The drawing under review shows one solid part. Ordinate dimensions are in mm from its lowest x, y, z. A direction names the side the tool comes from. Coordinates: 2 decimals unless noted, no trailing zeros. Order: outer loops, then holes, each group sorted by start corner. A loop starts at its lowest first (then second) coordinate and runs counter-clockwise, first axis right, second up. Notation, with made-up numbers: (62.5, 13.5) -> (118.5, 13.5) arc R26 cw to (118.5, 52.5) -> close; hole circle Ø10 at (67, -38). An arc over 180 degrees is marked (long way). Write item = value, one per line.
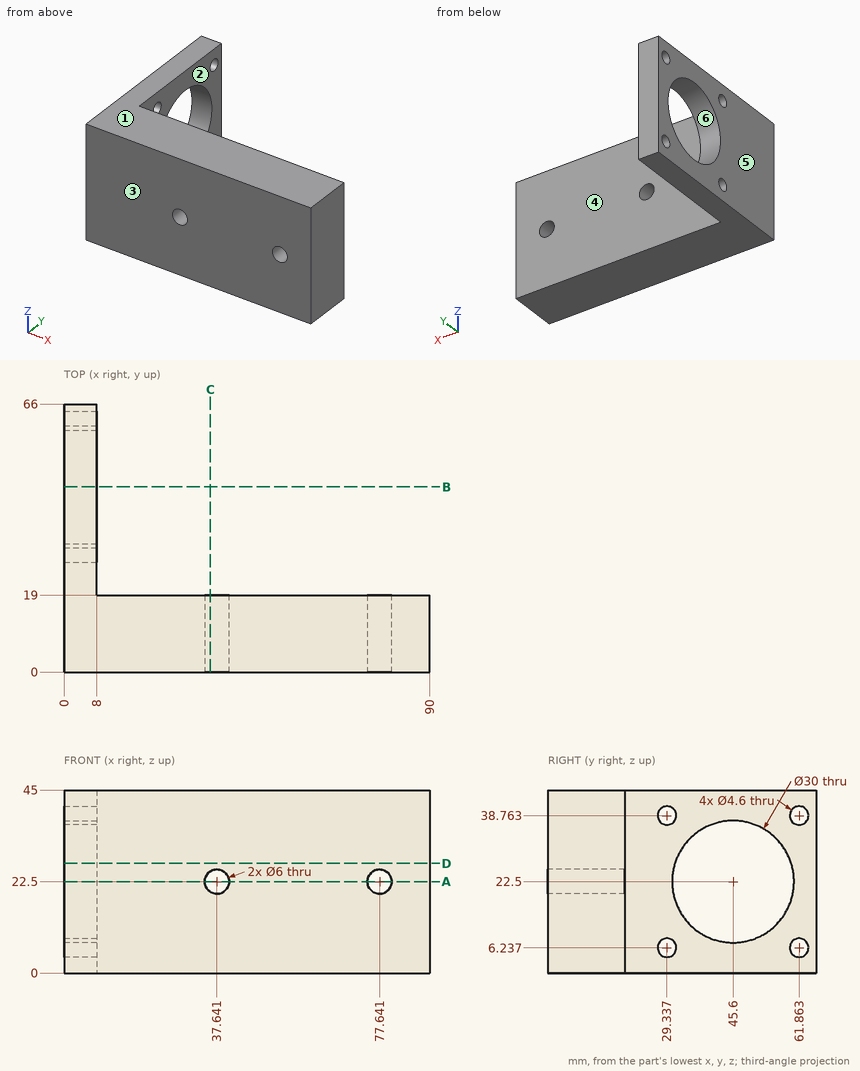
(1) For the marked faces 1 and 2, list the 3-axis set-ups (+Z, -Z, +X, -X, +Y, -Y) from which the entire face can be reached by the end or side of a thin tool; tool diameter is ignored.
Report:
face_1 = +Z, +X, -X, +Y, -Y
face_2 = +Z, -Z, +X, +Y
(2) We need section C-C (x = 36). Write out the cut boundary in (y, z).
Report:
outline = (0, 0) -> (19, 0) -> (19, 19.99) -> (0, 19.99) -> close; (0, 25.01) -> (19, 25.01) -> (19, 45) -> (0, 45) -> close
(3) We need section D-D (z = 27). Write out the cut boundary in (x, y).
Report:
outline = (0, 0) -> (90, 0) -> (90, 19) -> (8, 19) -> (8, 31.29) -> (0, 31.29) -> close; (0, 59.91) -> (8, 59.91) -> (8, 66) -> (0, 66) -> close
(4) We need section B-B (y = 45.6). Write out the cut boundary in (x, z).
Report:
outline = (0, 0) -> (8, 0) -> (8, 7.5) -> (0, 7.5) -> close; (0, 37.5) -> (8, 37.5) -> (8, 45) -> (0, 45) -> close
(5) For L1, parallel to X at y = 12, z = 21.5; L2, parallel to X at y = 11, z = 22; L3, parallel to Y at x = 20, z = 16, list the stretches that pass through material, from the lowest coordinate up.
Report:
L1 = 0 to 34.81, 40.47 to 74.81, 80.47 to 90
L2 = 0 to 34.68, 40.6 to 74.68, 80.6 to 90
L3 = 0 to 19
(6) Insertion check: pin 1 (1.5 mm diameter, centred on x = 31, z = 13.5, fed in from -Y); pin 2 (8 mm diameter, centred on x = 17.5, z = 33.5, fed in from +Y); pin 3 (3.5 mm diameter, centred on y = 61.86, z = 6.24, fed in from -X) (1 decimal); pin 4 (10 mm diameter, centred on y = 35, z = 22.5, fed in from +X). Each pin has a flat end and moves straight along its axis. Give the tip position at first contact, or say it passes through.
Report:
pin_1 = 0
pin_2 = 19
pin_3 = through
pin_4 = 8
(7) The part is to be moulded in two halves that separate along Y. For the marked faces 3, 4, 5 and 6, say which applies: released by +Y, released by -Y, zero draft, split by the parting line, or undercut.
Report:
face_3 = released by -Y
face_4 = released by +Y
face_5 = zero draft
face_6 = undercut
(8) We need section A-A (z = 22.5). Write out the cut boundary in (x, y).
Report:
outline = (0, 0) -> (34.64, 0) -> (34.64, 19) -> (8, 19) -> (8, 30.6) -> (0, 30.6) -> close; (0, 60.6) -> (8, 60.6) -> (8, 66) -> (0, 66) -> close; (40.64, 0) -> (74.64, 0) -> (74.64, 19) -> (40.64, 19) -> close; (80.64, 0) -> (90, 0) -> (90, 19) -> (80.64, 19) -> close
